```python
from build123d import *

# Parameters (mm, degrees)
F0_W     = 38.1
F0_H     = 38.1
F1_DEPTH = 0.79375
F2_W     = 38.1
F2_H     = 38.1
F2_W_2   = 34.925
F2_H_2   = 34.925
F3_DEPTH = 5.08
F4_W     = 23.495
F4_H     = 1.7271855524
F4_W_2   = 1.9184793842
F4_H_2   = 10.6553144476
F4_W_3   = 16.4965206158
F4_H_3   = 1.27
F4_W_4   = 15.3910815895
F4_H_4   = 0.9525
F5_DEPTH = 4.445
F4_R     = 1.27
F6_DEPTH = 0.396875


with BuildPart() as f1:
    # F0 (on Top) → F1 (new body)
    with BuildSketch(Plane.XY):
        with Locations((-5.3514037281, -3.4365521467)):
            Rectangle(F0_W, F0_H)
    extrude(amount=F1_DEPTH)

    # F2 (on face) → F3 (join)
    with BuildSketch(Plane.XY.offset(0.79375)):
        with Locations((-5.3514037281, -3.4365521467)):
            Rectangle(F2_W, F2_H)
        with Locations((-5.3514037281, -3.4365521467)):
            Rectangle(F2_W_2, F2_H_2, mode=Mode.SUBTRACT)
    extrude(amount=F3_DEPTH)

    # F4 (on face) → F5 (join)
    with BuildSketch(Plane.XY.offset(0.79375)):
        Polygon((-17.7339037281, 8.9459478533), (-17.7339037281, -20.8990521467), (-16.4639037281, -20.8990521467), (-16.4639037281, -9.7865521467), (-16.4639037281, -8.5165521467), (-16.4639037281, 7.2187623009), (-16.4639037281, 8.9459478533), align=None)
        with Locations((-4.7164037281, 8.0823550771)):
            Rectangle(F4_W, F4_H)
        with Locations((-10.424664036, -3.1888949229)):
            Rectangle(F4_W_2, F4_H_2)
        Polygon((-16.4639037281, -8.5165521467), (-16.4639037281, -9.7865521467), (-9.4654243439, -9.7865521467), (-9.4654243439, -8.5165521467), (-11.3839037281, -8.5165521467), align=None)
        Polygon((-9.4654243439, -8.5165521467), (-9.4654243439, -9.7865521467), (5.7610962719, -9.7865521467), (7.0310962719, -9.7865521467), (7.0310962719, -8.5165521467), align=None)
        with Locations((3.862835964, -2.8015521467)):
            Rectangle(F4_W_3, F4_H_3)
        Polygon((7.0310962719, -9.7865521467), (5.7610962719, -9.7865521467), (5.7610962719, -14.8665521467), (5.7610962719, -15.8190521467), (7.0310962719, -15.8190521467), align=None)
        with Locations((-1.9344445229, -15.3428021467)):
            Rectangle(F4_W_4, F4_H_4)
    extrude(amount=F5_DEPTH)

    # F4 (on face) → F6 (cut)
    with BuildSketch(Plane.XY.offset(0.79375)):
        with Locations((-20.5732807517, -14.9969505146)):
            Circle(F4_R)
        with Locations((-14.5668098703, -18.4527281672)):
            Circle(F4_R)
    extrude(amount=-F6_DEPTH, mode=Mode.SUBTRACT)


solid = f1.part
```
The model under review builds one solid part; all positions refer to its coordinate system, in mm. A direction names the side the tool comes from. Coordinates: 2 decimals unless noted, no trailing zeros. Loops run counter-clockwise (first coordinate to the right, second up) from the corner with the lowest first, then second, coordinate; pieces in that order, holes last. Notation, with made-up numbers: (-21.75, 85.25) -> (-7.75, 85.25) arc R23 ccw to (-7.75, 110.25) -> close; hole circle Ø2 at (58, -34.5). An arc over 180 degrees is marked (long way). Answer as CSV lines item,"result".
Item 1: Take a section at C-C, the plane y = -13. State the section outline as (x, z) points, and give its area (3 significant figures).
Results below:
outline,"(-24.4, 0) -> (13.7, 0) -> (13.7, 5.87) -> (12.11, 5.87) -> (12.11, 0.79) -> (7.03, 0.79) -> (7.03, 5.24) -> (5.76, 5.24) -> (5.76, 0.79) -> (-16.46, 0.79) -> (-16.46, 5.24) -> (-17.73, 5.24) -> (-17.73, 0.79) -> (-22.81, 0.79) -> (-22.81, 5.87) -> (-24.4, 5.87) -> close"
area,"57.7 mm2"
Item 2: Take a section at D-D, the plane x = -3. State the section outline as (y, z) points.
Results below:
outline,"(-22.49, 0) -> (15.61, 0) -> (15.61, 5.87) -> (14.03, 5.87) -> (14.03, 0.79) -> (8.95, 0.79) -> (8.95, 5.24) -> (7.22, 5.24) -> (7.22, 0.79) -> (-2.17, 0.79) -> (-2.17, 5.24) -> (-3.44, 5.24) -> (-3.44, 0.79) -> (-8.52, 0.79) -> (-8.52, 5.24) -> (-9.79, 5.24) -> (-9.79, 0.79) -> (-14.87, 0.79) -> (-14.87, 5.24) -> (-15.82, 5.24) -> (-15.82, 0.79) -> (-20.9, 0.79) -> (-20.9, 5.87) -> (-22.49, 5.87) -> close"
Item 3: For L1, parallel to X at y = -15, z = 1.05; L2, parallel to X at y = -7, z = 1; L3, parallel to Y at x = -8, z = 4.15, list the stretches that pass through material, from the lowest coordinate up.
Results below:
L1,"x = -24.4 to -22.81, -17.73 to -16.46, -9.63 to 7.03, 12.11 to 13.7"
L2,"x = -24.4 to -22.81, -17.73 to -16.46, -11.38 to -9.47, 12.11 to 13.7"
L3,"y = -22.49 to -20.9, -15.82 to -14.87, -9.79 to -8.52, 7.22 to 8.95, 14.03 to 15.61"
Item 4: Take a section at B-B, the plane x = 8. State the section outline as (y, z) points, and give its area (3 significant figures).
Results below:
outline,"(-22.49, 0) -> (15.61, 0) -> (15.61, 5.87) -> (14.03, 5.87) -> (14.03, 0.79) -> (-2.17, 0.79) -> (-2.17, 5.24) -> (-3.44, 5.24) -> (-3.44, 0.79) -> (-20.9, 0.79) -> (-20.9, 5.87) -> (-22.49, 5.87) -> close"
area,"52.0 mm2"
Item 5: Draft analysis for pull direction X (two halves, no side actions). For faces 1 (the flat face through (13.699, -4, 3)), 2 (the flat face through (-7, -22, 5.874)), 3 (the flat face through (-21, -15, 0.397)), state which applies: +X half, -X half, draft (parallel to the pull), parting line (faces both ways), or undercut.
Results below:
face 1,"+X half"
face 2,"draft"
face 3,"undercut"
Item 6: Insertion check: pin 1 (6 mm diameter, centred on x = -9.5, y = -1.5, fed in from +Z); pin 2 (0.8 mm diameter, centred on x = -20.5, y = -15, fed in from +Z). Each pin has a flat end and moves straight along its axis. Give the tip position at first contact, or say it passes through.
Results below:
pin 1,"stops at z = 5.24"
pin 2,"stops at z = 0.4"
Item 7: Machinability: for faces 4 (the flat face through (-17.734, -6, 3)), 5 (the flat face through (-24.401, -4, 3)), which of the approach directions +Z, -Z, +X, -X, +Y, -Y give a long, thin tool a straight path to every point of the face, cutting with its end or side? Answer none if there is none.
Results below:
face 4,"+Z"
face 5,"+Z, -Z, -X, +Y, -Y"
